```python
from build123d import *

# Parameters (mm, degrees)
PAD_DEPTH     = 10
SKETCH002_R   = 2.85
POCKET_DEPTH  = 30
SKETCH003_R   = 3.5
SKETCH003_R_2 = 1.643
PAD001_DEPTH  = 2


with BuildPart() as part:
    # Sketch → Pad (new body)
    with BuildSketch(Plane.XZ):
        Polygon((0, 0), (0, 1), (70, 13.342889), (70, 0), align=None)
    extrude(amount=PAD_DEPTH)

    # Sketch002 (on Face4 of Pad) → Pocket (cut)
    with BuildSketch(Plane(origin=(0, 0, 0), x_dir=(1, 0, 0), z_dir=(0, 0, -1))):
        with Locations((32, 5)):
            Circle(SKETCH002_R)
        with Locations((62, 5)):
            Circle(SKETCH002_R)
    extrude(amount=-POCKET_DEPTH, mode=Mode.SUBTRACT)

    # Sketch003 (on Face2 of Pocket) → Pad001 (join)
    with BuildSketch(Plane(origin=(0, 0, 0), x_dir=(1, 0, 0), z_dir=(0, 0, -1))):
        with Locations((32, 5)):
            Circle(SKETCH003_R)
        with Locations((32, 5)):
            Circle(SKETCH003_R_2, mode=Mode.SUBTRACT)
        with Locations((62, 5)):
            Circle(SKETCH003_R)
        with Locations((62, 5)):
            Circle(SKETCH003_R_2, mode=Mode.SUBTRACT)
    extrude(amount=-PAD001_DEPTH)


solid = part.part
```
Part model, mm, in its own coordinate system. A direction names the side the tool comes from. Coordinates: 2 decimals unless noted, no trailing zeros. Order: outer loops, then holes, each group sorted by start corner. A loop starts at its lowest first (then second) coordinate and runs counter-clockwise, first axis right, second up. Notation, with made-up numbers: (-1, -25.5) - (15, -25.5) arc R18 ccw to (15, -10.5) - close; hole circle Ø8 at (24, 20). An arc over 180 degrees is marked (long way). Return JSON: item names as keys, results as strings. Group by question number.
Item 1: Cut at D-D (z = 3). List the corners of the cut face in (x, y), plus the area to 3 significant figures.
Item 2: Pull direction X, two halves, no side cores. Call faces 1 (the face through (33.57, -5.49, 0.99)), 2 (the face through (43, 0, 5)), 3 (the face through (70, -5, 7)): pulls with the +X half, pulls with the -X half, needs draft (parallel to the pull), parting line crosses it, or undercut.
Item 3: Cut at A-A (y = -5). List the corners of the cut face in (x, z) (3 decimals), plus the area to 3 significant figures.
Item 4: Cut at B-B (x = 62). List the corners of the cut face in (y, z).
Item 5: Which spindle directions (+Z, -Z, +X, -X, +Y, -Y) get a long thin tool onto all of the face, cutting with end or side? Do faces 4 (the face through (35, -5, 0)), 5 (the face through (34, -5, 2)). Say none if no direction does.
Item 6: Pin check, flat tips, straight feed: pin 1 (2 mm diameter, centred on x = 63, y = -4, fed in from +Z); pin 2 (4.5 mm diameter, centred on x = 62.5, y = -4.5, fed in from +Z); pin 3 (5 mm diameter, centred on x = 36, y = -6, fed in from +Z). Stop position of each tip, or through.
Item 7: Cut at C-C (z = 8). List the corners of the cut face in (x, y).
Item 8: Drill centre lines: probe 1 along X at (y, z) = (-5, 0.6); probe 2 along Y at (x, z) = (62, 6.5); probe 3 along Z at (x, y) = (6, -1.25). Where is each one in solid material? Low to high. Write a range as from..to.
Check values:
{
 "1": {"outline": "(11.34, -10) - (70, -10) - (70, 0) - (11.34, 0) - close; hole circle Ø5.7 at (32, -5); hole circle Ø5.7 at (62, -5)", "area": "536 mm2"},
 "2": {"face 1": "undercut", "face 2": "needs draft", "face 3": "pulls with the +X half"},
 "3": {"outline": "(0, 0) - (30.357, 0) - (30.357, 2) - (29.15, 2) - (29.15, 6.14) - (0, 1) - close; (33.643, 0) - (60.357, 0) - (60.357, 2) - (59.15, 2) - (59.15, 11.43) - (34.85, 7.145) - (34.85, 2) - (33.643, 2) - close; (63.643, 0) - (70, 0) - (70, 13.343) - (64.85, 12.435) - (64.85, 2) - (63.643, 2) - close", "area": "406 mm2"},
 "4": {"outline": "(-10, 0) - (-6.64, 0) - (-6.64, 2) - (-7.85, 2) - (-7.85, 11.93) - (-10, 11.93) - close; (-3.36, 0) - (0, 0) - (0, 11.93) - (-2.15, 11.93) - (-2.15, 2) - (-3.36, 2) - close"},
 "5": {"face 4": "-Z, +X, -X, +Y, -Y", "face 5": "+Z"},
 "6": {"pin 1": "stops at z = 2", "pin 2": "stops at z = 12.41", "pin 3": "stops at z = 7.79"},
 "7": {"outline": "(39.7, -10) - (70, -10) - (70, 0) - (39.7, 0) - close; hole circle Ø5.7 at (62, -5)"},
 "8": {"probe 1": "x = 0..30.36, 33.64..60.36, 63.64..70", "probe 2": "y = -10..-7.85, -2.15..0", "probe 3": "z = 0..2.06"}
}
